```python
from build123d import *

# Parameters (mm, degrees)
F1_DEPTH     = 1.5
F3_DEPTH     = 5
F4_T         = 1.5
F4_T3_DEPTH  = 4.5
F4_T5_DEPTH  = 10.4166599398
F4_T7_DEPTH  = 10
F4_T9_DEPTH  = 25
F4_T11_DEPTH = 24
F4_T13_DEPTH = 34.9687469041
F4_T15_DEPTH = 53.4166599398
F4_T17_DEPTH = 8


# Not quite as in the source:
# - a shell that OpenCascade refuses in one call is made with other operations: the cavity is built on its own and cut out


with BuildPart() as f1:
    # F0 (on Front) → F1 (new body)
    with BuildSketch(Plane.XZ):
        Polygon((-52.3250011176, 25.3536881179), (-52.3250011176, -14.8463118821), (7.8749988824, -14.8463118821), (7.8749988824, 25.3536881179), (1.8749988824, 25.3536881179), (1.8749988824, 34.3536881179), (-32.1250011176, 34.3536881179), (-32.1250011176, 25.3536881179), align=None)
    extrude(amount=F1_DEPTH)

    # F2 (on face) → F3 (join)
    with BuildSketch(Plane.XZ.offset(1.5)):
        Polygon((-46.9777897949, 21.0005849694), (-46.9777897949, -10.9681619347), (3.4388701449, -10.9681619347), (3.4388701449, 21.0005849694), (-3.9777897949, 21.0005849694), (-3.9777897949, 28.0005849694), (-25.9777897949, 28.0005849694), (-25.9777897949, 21.0005849694), align=None)
    extrude(amount=F3_DEPTH)

    # F4: shell of thickness 1.5, made by hand


with BuildPart() as f4_core1:
    # F4_t2: copy of F1
    add(f1.part)

    # the walls: a layer under each face that stays
    f4_faces = [f4_core1.faces().sort_by_distance(p)[0] for p in [
        (-42.2250011176, -0.75, 25.3536881179),
        (-32.1250011176, -0.75, 29.8536881179),
        (-52.3250011176, -0.75, 5.2536881179),
        (-22.2250011176, 0, 9.7536881179),
        (-2.1583344509, -1.5, 26.1536881179),
        (-15.1250011176, -0.75, 34.3536881179),
        (-22.2250011176, -0.75, -14.8463118821),
        (7.8749988824, -0.75, 5.2536881179),
        (4.8749988824, -0.75, 25.3536881179),
        (1.8749988824, -0.75, 29.8536881179),
        (-0.269459825, -4, 21.0005849694),
        (-3.9777897949, -4, 24.5005849694),
        (-14.9777897949, -4, 28.0005849694),
        (-25.9777897949, -4, 24.5005849694),
        (-36.4777897949, -4, 21.0005849694),
        (-46.9777897949, -4, 5.0162115173),
        (-21.769459825, -4, -10.9681619347),
        (3.4388701449, -4, 5.0162115173),
    ]]
    thicken(f4_faces, amount=-F4_T, mode=Mode.SUBTRACT)

    # F4_s4 → F4_t3 (cut)
    with BuildSketch(Plane.XZ.offset(-1.5)):
        Polygon((-32.1400011176, 25.3686881179), (-32.1250011176, 23.8536881179), (-30.6250011176, 23.8536881179), (-30.6250011176, 25.3536881179), align=None)
        Polygon((1.8899988824, 25.3686881179), (1.8749988824, 23.8536881179), (0.3749988824, 23.8536881179), (0.3749988824, 25.3536881179), align=None)
    extrude(amount=F4_T3_DEPTH, mode=Mode.SUBTRACT)

    # F4_s6 → F4_t5 (cut)
    with BuildSketch(Plane.YZ.offset(-5.4777897949)):
        Polygon((-1.515, 21.0155849694), (0, 21.0005849694), (0, 19.5005849694), (-1.5, 19.5005849694), align=None)
    extrude(amount=F4_T5_DEPTH, mode=Mode.SUBTRACT)

    # F4_s8 → F4_t7 (cut)
    with BuildSketch(Plane.XY.offset(19.5005849694)):
        Polygon((-3.9627897949, -1.515), (-3.9777897949, 0), (-5.4777897949, 0), (-5.4777897949, -1.5), align=None)
        Polygon((-25.9927897949, -1.515), (-25.9777897949, 0), (-24.4777897949, 0), (-24.4777897949, -1.5), align=None)
    extrude(amount=F4_T7_DEPTH, mode=Mode.SUBTRACT)

    # F4_s10 → F4_t9 (cut)
    with BuildSketch(Plane.YZ.offset(-27.4777897949)):
        Polygon((-1.515, 28.0155849694), (0, 28.0005849694), (0, 26.5005849694), (-1.5, 26.5005849694), align=None)
    extrude(amount=F4_T9_DEPTH, mode=Mode.SUBTRACT)

    # F4_s12 → F4_t11 (cut)
    with BuildSketch(Plane.YZ.offset(-48.4777897949)):
        Polygon((-1.515, 21.0155849694), (0, 21.0005849694), (0, 19.5005849694), (-1.5, 19.5005849694), align=None)
    extrude(amount=F4_T11_DEPTH, mode=Mode.SUBTRACT)

    # F4_s14 → F4_t13 (cut)
    with BuildSketch(Plane.XY.offset(-12.4681619347)):
        Polygon((-46.9927897949, -1.515), (-46.9777897949, 0), (-45.4777897949, 0), (-45.4777897949, -1.5), align=None)
        Polygon((3.4538701449, -1.515), (3.4388701449, 0), (1.9388701449, 0), (1.9388701449, -1.5), align=None)
    extrude(amount=F4_T13_DEPTH, mode=Mode.SUBTRACT)

    # F4_s16 → F4_t15 (cut)
    with BuildSketch(Plane.YZ.offset(-48.4777897949)):
        Polygon((-1.515, -10.9831619347), (0, -10.9681619347), (0, -9.4681619347), (-1.5, -9.4681619347), align=None)
    extrude(amount=F4_T15_DEPTH, mode=Mode.SUBTRACT)

    # F4_s18 → F4_t17 (cut)
    with BuildSketch(Plane.XZ):
        Polygon((-3.9627897949, 21.0155849694), (-3.9777897949, 19.5005849694), (-5.4777897949, 19.5005849694), (-5.4777897949, 21.0005849694), align=None)
        Polygon((-25.9927897949, 21.0155849694), (-24.4777897949, 21.0005849694), (-24.4777897949, 19.5005849694), (-25.9777897949, 19.5005849694), align=None)
    extrude(amount=F4_T17_DEPTH, mode=Mode.SUBTRACT)


with BuildPart() as f1_1:
    add(f1.part)

    # what is left inside the walls is the cavity
    f4_cavity = [f4_core1.part.solids().sort_by_distance(p)[0] for p in [
        (-21.76946, -1.515, 2.52142),
    ]]
    add(f4_cavity, mode=Mode.SUBTRACT)


solid = f1_1.part
```
Model file for the job. Use its own axes, mm. A direction names the side the tool comes from. Give positions to 0.01 mm unless a question says otherwise; leave off trailing zeros. Loops run counter-clockwise (first coordinate to the right, second up) from the corner with the lowest first, then second, coordinate; pieces in that order, holes last. Notation, with made-up numbers: (84, -38.75) -> (136, -38.75) arc R7 cw to (136, -34.75) -> close; hole circle Ø6 at (53.25, 62). An arc over 180 degrees is marked (long way). Use CSV: the item, a comma, the result in double quotes. Start each with the question number.
1) Slice it at C-C on z = -4. Give the cut face in (x, y) (3 decimals).
2) Slice it at B-B on x = -43.5. Give the cut face in (y, z), plus the area to 3 significant figures.
3) Slice it at A-A on y = -5.5. Give the cut face in (x, z), plus the area to 3 significant figures.
4) Flat gauge pins, fed straight in: pin 1 Ø1.2 at (x, y) = (4, -1) entering from +Z; pin 2 Ø2.5 at (x, y) = (0.5, -5) entering from +Z; pin 3 Ø6 at (x, z) = (-34.5, 15.5) entering from -Y. Where does each tip first touch, or does it go through?
5) Slice it at D-D on y = -0.75. Give the cut face in (x, z) (3 decimals).
6) Wall check: line 1 (X direction, y = -6, z = 9); line 2 (Z direction, x = 1, y = -4.5); line 3 (Z direction, x = -13.5, y = -2). Give the ranges that are in metal, low to high.
7) Mould opens along Z. For faces 5 (the flat face through (-42, -1, 25.354)), 6 (the flat face through (-29, -1.5, 26)), 7 (the flat face through (-45.478, -4, 5)) say: released by +Z, released by -Z, zero draft, split by the parting line, or undercut.
8) Tool access for faces 1 (the flat face through (-2, -4, 19.501)), 2 (the flat face through (0, -4, 21.001)), 3 (the flat face through (-15, -4, 28.001)), 4 (the flat face through (-22, -4, -10.968)): list every direction of +Z, -Z, +X, -X, +Y, -Y with a clear straight run to the whole face (end or side of a thin tool).
Computed values:
1,outline,"(-52.325, -1.5) -> (-46.978, -1.5) -> (-46.978, -6.5) -> (-45.478, -6.5) -> (-45.478, -1.5) -> (1.939, -1.5) -> (1.939, -6.5) -> (3.439, -6.5) -> (3.439, -1.5) -> (7.875, -1.5) -> (7.875, 0) -> (-52.325, 0) -> close"
2,outline,"(-6.5, -10.97) -> (-1.5, -10.97) -> (-1.5, -14.85) -> (0, -14.85) -> (0, 25.35) -> (-1.5, 25.35) -> (-1.5, 21) -> (-6.5, 21) -> (-6.5, 19.5) -> (-1.5, 19.5) -> (-1.5, -9.47) -> (-6.5, -9.47) -> close"
2,area,"75.3 mm^2"
3,outline,"(-46.98, -10.97) -> (3.44, -10.97) -> (3.44, 21) -> (-3.98, 21) -> (-3.98, 28) -> (-25.98, 28) -> (-25.98, 21) -> (-46.98, 21) -> close; hole (-45.48, -9.47) -> (1.94, -9.47) -> (1.94, 19.5) -> (-5.48, 19.5) -> (-5.48, 26.5) -> (-24.48, 26.5) -> (-24.48, 19.5) -> (-45.48, 19.5) -> close"
3,area,"259 mm^2"
4,pin 1,"stops at z = 25.35"
4,pin 2,"stops at z = 21"
4,pin 3,"stops at y = -1.5"
5,outline,"(-52.325, -14.846) -> (7.875, -14.846) -> (7.875, 25.354) -> (1.875, 25.354) -> (1.875, 34.354) -> (-32.125, 34.354) -> (-32.125, 25.354) -> (-52.325, 25.354) -> close"
6,line 1,"x = -46.98 to -45.48, 1.94 to 3.44"
6,line 2,"z = -10.97 to -9.47, 19.5 to 21"
6,line 3,"z = -10.97 to -9.47, 26.5 to 28"
7,face 5,"released by +Z"
7,face 6,"zero draft"
7,face 7,"undercut"
8,face 1,"-Y"
8,face 2,"+Z, +X, -Y"
8,face 3,"+Z, +X, -X, -Y"
8,face 4,"-Z, +X, -X, -Y"
